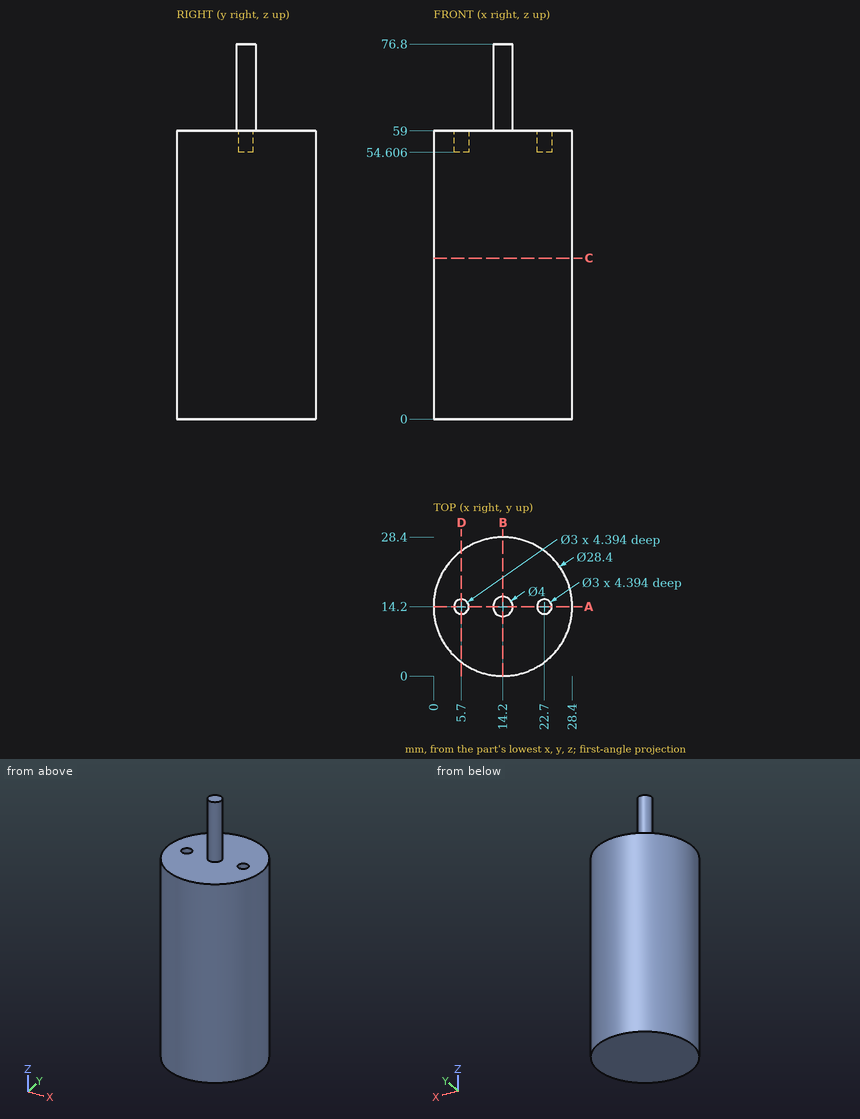
Could you check a few things on this drawing? It's one solid part, dimensions in mm from its lowest x, y, z. Coordinates: 2 decimals unless noted, no trailing zeros. Order: outer loops, then holes, each group sorted by start corner. A loop starts at its lowest first (then second) coordinate and runs counter-clockwise, first axis right, second up. Notation, with made-up numbers: (4.25, 7) -> (55.25, 7) arc R18 cw to (55.25, 18) -> close; hole circle Ø1 at (-8.75, 84.25). An arc over 180 degrees is marked (long way). One line per item, written item: value. Start each with the question number.
1) Imagine slicing it at B-B on x = 14.2. List the corners of the cut face in (y, z) for me.
2) If I drill on L1, parallel to Z at x = 10, y = 16; L2, parallel to Y at x = 5.7, z = 57.8 (1 decimal); L3, parallel to Z at x = 24, y = 14, over which ranges is the centre line in solid material (lowest first)? Write a range as [from, to].
3) Imagine slicing it at C-C on z = 33. List the corners of the cut face in (x, y) for me.
4) Imagine slicing it at A-A on y = 14.2. List the corners of the cut face in (x, z) for me.
5) Imagine slicing it at D-D on x = 5.7. List the corners of the cut face in (y, z) for me (1 decimal), plus the area to 3 significant figures.
6) I'm going to push flat-ended pins straight in: pin 1 (0.9 mm diameter, centred on x = 6, y = 15, fed in from +Z); pin 2 (2.5 mm diameter, centred on x = 22.7, y = 14.2, fed in from -Z); pin 3 (6 mm diameter, centred on x = 20.5, z = 18.5, fed in from -Y); pin 4 (8 mm diameter, centred on x = 20, y = 18.5, fed in from +Z). Where does each tip first touch, or does it pass through?
Answer list:
1. outline: (0, 0) -> (28.4, 0) -> (28.4, 59) -> (16.2, 59) -> (16.2, 76.8) -> (12.2, 76.8) -> (12.2, 59) -> (0, 59) -> close
2. L1: z = [0, 59]
2. L2: y = [2.8, 12.7], [15.7, 25.6]
2. L3: z = [0, 54.61]
3. outline: circle Ø28.4 at (14.2, 14.2)
4. outline: (0, 0) -> (28.4, 0) -> (28.4, 59) -> (24.2, 59) -> (24.2, 54.61) -> (21.2, 54.61) -> (21.2, 59) -> (16.2, 59) -> (16.2, 76.8) -> (12.2, 76.8) -> (12.2, 59) -> (7.2, 59) -> (7.2, 54.61) -> (4.2, 54.61) -> (4.2, 59) -> (0, 59) -> close
5. outline: (2.8, 0) -> (25.6, 0) -> (25.6, 59) -> (15.7, 59) -> (15.7, 54.6) -> (12.7, 54.6) -> (12.7, 59) -> (2.8, 59) -> close
5. area: 1,330 mm2
6. pin 1: stops at z = 54.61
6. pin 2: stops at z = 0
6. pin 3: stops at y = 0.39
6. pin 4: stops at z = 59
